from build123d import *

# Parameters (mm, degrees)
SKETCH1_R           = 27.5
BOSS_EXTRUDE1_DEPTH = 29
SKETCH2_R           = 25.5
SKETCH2_R_2         = 5
CUT_EXTRUDE1_DEPTH  = 26
CUT_EXTRUDE2_DEPTH  = 26
SKETCH4_R           = 5
CUT_EXTRUDE3_DEPTH  = 16
CHAMFER1_SIZE       = 1


with BuildPart() as part:
    # Sketch1 → Boss-Extrude1 (new body)
    with BuildSketch(Plane.XY):
        with Locations(Location((0, 0, 0), (0, 0, 180))):
            Circle(SKETCH1_R)
    extrude(amount=BOSS_EXTRUDE1_DEPTH)

    # Sketch2 → Cut-Extrude1 (cut)
    with BuildSketch(Plane.XY.offset(29)):
        Circle(SKETCH2_R)
        Circle(SKETCH2_R_2, mode=Mode.SUBTRACT)
    extrude(amount=-CUT_EXTRUDE1_DEPTH, mode=Mode.SUBTRACT)

    # Sketch3 → Cut-Extrude2 (cut)
    with BuildSketch(Plane.XY.offset(29)):
        with BuildLine():
            Line((0.71010636, 3.017573356), (3.099332288, 0.064337932))
            ThreePointArc((3.099332288, 0.064337932), (-2.410053022, -1.949780611), (0.71010636, 3.017573356))
        make_face()
    extrude(amount=-CUT_EXTRUDE2_DEPTH, mode=Mode.SUBTRACT)

    # Sketch4 → Cut-Extrude3 (cut)
    with BuildSketch(Plane.XY.offset(29)):
        Circle(SKETCH4_R)
    extrude(amount=-CUT_EXTRUDE3_DEPTH, mode=Mode.SUBTRACT)

    # Chamfer1
    chamfer1_edges = [part.edges().sort_by_distance(p)[0] for p in [
        (27.5, 0, 0),
    ]]
    chamfer(chamfer1_edges, length=CHAMFER1_SIZE)


solid = part.part
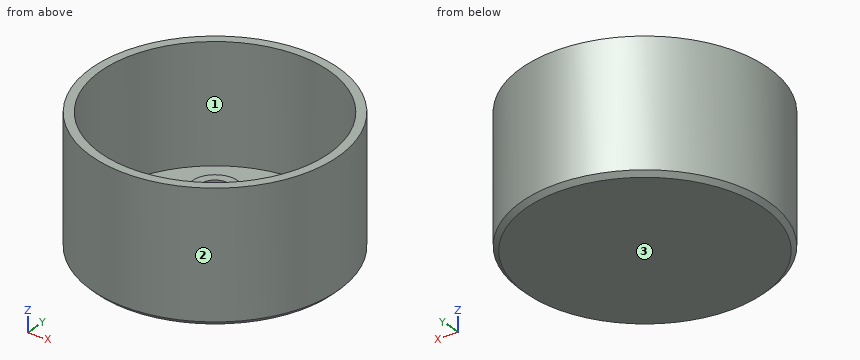
Read the model definition and answer for the solid it produces. Units are mm, in the model's axes. Face numbers are marked on the shaded views. Give positions to 0.01 mm unless a question says otherwise; leave off trailing zeros. Loops run counter-clockwise (first coordinate to the right, second up) from the corner with the lowest first, then second, coordinate; pieces in that order, holes last. Notation, with made-up numbers: (-37.5, -17.5) -> (-3.5, -17.5) arc R16 cw to (-3.5, -3.5) -> close; hole circle Ø6 at (-0.75, -24). An arc over 180 degrees is marked (long way). Answer as CSV lines item,"result".
Item 1: Find section B-B on x = 0. Give the vertices of the cut face in (y, z), plus the area to 3 significant figures.
Returned:
outline,"(-27.5, 1) -> (-26.5, 0) -> (26.5, 0) -> (27.5, 1) -> (27.5, 29) -> (25.5, 29) -> (25.5, 3) -> (5, 3) -> (5, 13) -> (3.1, 13) -> (3.1, 3) -> (-3.1, 3) -> (-3.1, 13) -> (-5, 13) -> (-5, 3) -> (-25.5, 3) -> (-25.5, 29) -> (-27.5, 29) -> close"
area,"306 mm²"
Item 2: Consider line 1 (Y direction, x = 0, z = 7.25); line 2 (Y direction, x = 0, z = 23.5); line 3 (Z direction, x = -2, y = 24.5). Determine where each line is inside the solid, lowest interval first. Write a range as [from, to].
Returned:
line 1,"y = [-27.5, -25.5], [-5, -3.1], [3.1, 5], [25.5, 27.5]"
line 2,"y = [-27.5, -25.5], [25.5, 27.5]"
line 3,"z = [0, 3]"
Item 3: Find section C-C on z = 15. Give the vertices of the cut face in (x, y), plus the area to 3 significant figures.
Returned:
outline,"circle Ø55 at (0, 0); hole circle Ø51 at (0, 0)"
area,"333 mm²"
Item 4: Find section A-A on z = 4.25. Give the vertices of the cut face in (x, y).
Returned:
outline,"circle Ø55 at (0, 0); circle Ø10 at (0, 0); hole circle Ø51 at (0, 0); hole (0.71, 3.02) arc R3.1 ccw (long way) to (3.1, 0.06) -> close"
Item 5: Each of these flat-tipped pins is pushed along its axis until it touches: pin 1 (1.5 mm diameter, centred on x = 20.5, y = -8.5, fed in from +Z); pin 2 (3 mm diameter, centred on x = -2.5, z = 3.5, fed in from -Y); pin 3 (8 mm diameter, centred on x = -1.5, y = -2, fed in from +Z); pin 4 (12 mm diameter, centred on x = 6, y = -19.5, fed in from +Z). Where does it stop, or does it pass through?
Returned:
pin 1,"stops at z = 3"
pin 2,"stops at y = -27.48"
pin 3,"stops at z = 13"
pin 4,"stops at z = 29"
Item 6: Determine the mould class of the marked faces 1, 2 and 3 for opening direction X: +X half, -X half, draft (parallel to the pull), parting line (faces both ways), or undercut.
Returned:
face 1,"undercut"
face 2,"parting line"
face 3,"draft"
